Input: part model. Units: mm. Frame: model coordinates. Face numbers are marked on the shaded views. Give positions to 0.01 mm unless a question says otherwise; leave off trailing zeros. Answer as a JSON object with one key per item and string values. Group by question number.
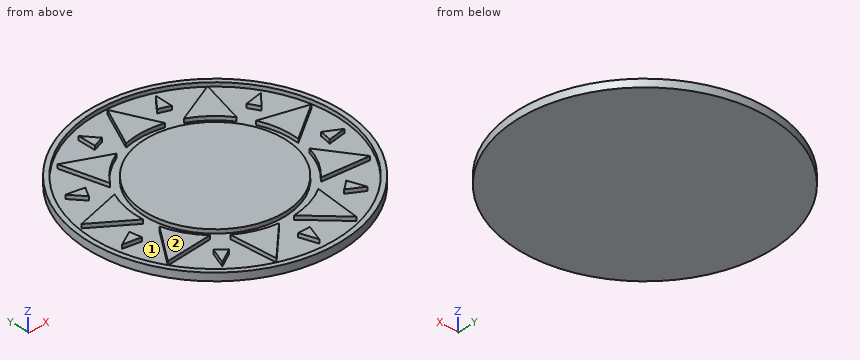
from build123d import *

# Parameters (mm, degrees)
F0_R     = 32.5
F1_DEPTH = 2
F2_R     = 31.3
F2_R_2   = 18
F3_DEPTH = 1
F5_DEPTH = 1
F6_COUNT = 9


with BuildPart() as f1:
    # F0 (on Top) → F1 (new body)
    with BuildSketch(Plane.XY):
        Circle(F0_R)
    extrude(amount=F1_DEPTH)

    # F2 (on face) → F3 (cut)
    with BuildSketch(Plane.XY.offset(2)):
        Circle(F2_R)
        Circle(F2_R_2, mode=Mode.SUBTRACT)
    extrude(amount=-F3_DEPTH, mode=Mode.SUBTRACT)

    # F4 (on face) → F5 (join, through all)
    with BuildSketch(Plane.XY.offset(1)):
        with BuildLine():
            ThreePointArc((-5, 19.364916731), (0, 20), (5, 19.364916731))
            add(Edge.make_bspline(
                [(0, 30), (5, 19.364916731), (0, 30), (5, 19.364916731)],
                knots=[0, 0, 0, 0, 11.7518082072, 11.7518082072, 11.7518082072, 11.7518082072], degree=3))
            add(Edge.make_bspline(
                [(-5, 19.364916731), (0, 30), (-5, 19.364916731), (0, 30)],
                knots=[0, 0, 0, 0, 11.7518082072, 11.7518082072, 11.7518082072, 11.7518082072], degree=3))
        make_face()
        with BuildLine():
            Line((9.8770545117, 22.7512776415), (9.9185841564, 27.2510860028))
            Line((9.9185841564, 27.2510860028), (7.0579766494, 23.7773380714))
            ThreePointArc((7.0579766494, 23.7773380714), (8.4830430925, 23.3069693448), (9.8770545117, 22.7512776415))
        make_face()
    extrude(amount=F5_DEPTH)

    # F6: F1 ×9 about axis
    f6_axis = Axis((0, 0, 0), (0, 0, -1))


with BuildPart() as f1_1:
    add(f1.part)
    for i in range(1, F6_COUNT):
        add(f1.part.rotate(f6_axis, i * 360 / F6_COUNT))


solid = f1_1.part
1) Mould query, pull axis Y, two halves, no side actions, for the marked faces 1 and 2. Classes: +Y half, -Y half, draft (parallel to the pull), parting line (faces both ways), or undercut.
2) Line query: line 1 along Y through (x, z) = (28, 1.25); line 2 along X through (y, z) = (0, 1.75); line 3 along Y through (x, z) = (14, 1.65). Output: solid intervals per line, ascending. Write a range as from..to.
3) Cut plane A-A on z = 1.4. Count the separate pieces of the cut face and the enclosed holes in it, and give its area (3 significant figures).
Filled in:
{
 "1": {"face 1": "undercut", "face 2": "draft"},
 "2": {"line 1": "y = -16.5..-13.99, -5.13..-4.72, 4.12..5.63, 13.99..16.5", "line 2": "x = -32.5..-31.3, -22.15..-20, -18..18, 20..22.15, 31.3..32.5", "line 3": "y = -29.33..-27.99, -11.31..11.31, 14.28..20.54, 27.99..29.33"},
 "3": {"separate pieces": "20", "enclosed holes": "1", "area": "1,760 mm²"}
}
